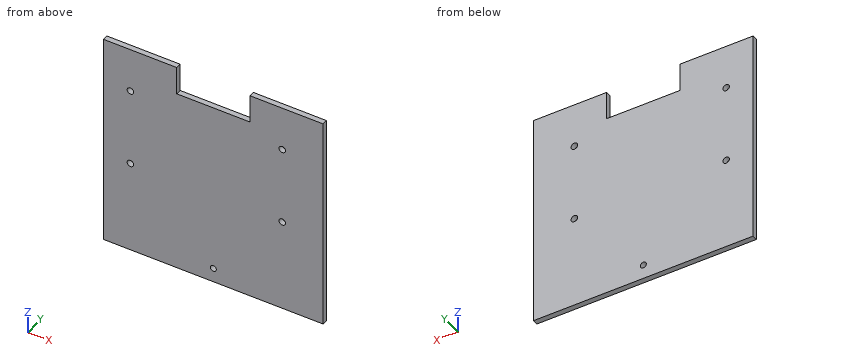
from build123d import *

# Parameters (mm, degrees)
SKETCH1_W           = 193.68
SKETCH1_H           = 190.5
BOSS_EXTRUDE1_DEPTH = 4.78
SKETCH2_R           = 2.6797
CUT_EXTRUDE1_DEPTH  = 5.78
CUT_EXTRUDE2_DEPTH  = 5.78
SKETCH4_R           = 2.893699953
CUT_EXTRUDE3_DEPTH  = 5.78


with BuildPart() as part:
    # Sketch1 → Boss-Extrude1 (new body)
    with BuildSketch(Plane(origin=(0, 0, 0), x_dir=(1, 0, 0), z_dir=(0, 1, 0))):
        Rectangle(SKETCH1_W, SKETCH1_H)
    extrude(amount=BOSS_EXTRUDE1_DEPTH)

    # Sketch2 → Cut-Extrude1 (cut, through all)
    with BuildSketch(Plane(origin=(0, 4.78, 0), x_dir=(1, 0, 0), z_dir=(0, 1, 0))):
        with Locations((0, 82.55)):
            Circle(SKETCH2_R)
    extrude(amount=-CUT_EXTRUDE1_DEPTH, mode=Mode.SUBTRACT)

    # Sketch3 → Cut-Extrude2 (cut, through all)
    with BuildSketch(Plane(origin=(0, 4.78, 0), x_dir=(1, 0, 0), z_dir=(0, 1, 0))):
        Polygon((0, -95.25), (-32.28, -95.25), (-32.28, -70.249999962), (32.28, -70.249999962), (32.28, -95.25), align=None)
    extrude(amount=-CUT_EXTRUDE2_DEPTH, mode=Mode.SUBTRACT)

    # Sketch4 → Cut-Extrude3 (cut, through all)
    with BuildSketch(Plane(origin=(0, 4.78, 0), x_dir=(1, 0, 0), z_dir=(0, 1, 0))):
        with Locations((-73.14, -55.899999962)):
            Circle(SKETCH4_R)
        with Locations((-73.14, 13.100000038)):
            Circle(SKETCH4_R)
        with Locations((60.86, 13.100000038)):
            Circle(SKETCH4_R)
        with Locations((60.86, -55.899999962)):
            Circle(SKETCH4_R)
    extrude(amount=-CUT_EXTRUDE3_DEPTH, mode=Mode.SUBTRACT)


solid = part.part
Input: part model. Units: mm. Frame: model coordinates. Coordinates: 2 decimals unless noted, no trailing zeros. Loops run counter-clockwise (first coordinate to the right, second up) from the corner with the lowest first, then second, coordinate; pieces in that order, holes last.
Q1. Contact query for a flat-ended pin moving along its axis: pin 1 (7 mm diameter, centred on x = 0, z = -82.55, fed in from -Y). Output: stop coordinate, or through.
Q2. Cut plane D-D (x = 0). Output: boundary loops of the cut face in (y, z).
Q3. Cut plane A-A (z = 55.9). Output: boundary loops of the cut face in (x, y).
Q4. Cut plane B-B (z = -82.55). Output: boundary loops of the cut face in (x, y).
Q5. Material intervals for line 1 (X direction, y = 3.05, z = 55.9); line 2 (Z direction, x = 60.86, y = 2.1); line 3 (Z direction, x = -71.5, y = 0.6), sorted ascending.
Q6. Cut plane C-C (y = 1.85). Output: boundary loops of the cut face in (x, z).
Working result:
1. pin 1: stops at y = 0
2. outline: (0, -95.25) - (4.78, -95.25) - (4.78, -85.23) - (0, -85.23) - close; (0, -79.87) - (4.78, -79.87) - (4.78, 70.25) - (0, 70.25) - close
3. outline: (-96.84, 0) - (-76.03, 0) - (-76.03, 4.78) - (-96.84, 4.78) - close; (-70.25, 0) - (57.97, 0) - (57.97, 4.78) - (-70.25, 4.78) - close; (63.75, 0) - (96.84, 0) - (96.84, 4.78) - (63.75, 4.78) - close
4. outline: (-96.84, 0) - (-2.68, 0) - (-2.68, 4.78) - (-96.84, 4.78) - close; (2.68, 0) - (96.84, 0) - (96.84, 4.78) - (2.68, 4.78) - close
5. line 1: x = -96.84 to -76.03, -70.25 to 57.97, 63.75 to 96.84
5. line 2: z = -95.25 to -15.99, -10.21 to 53.01, 58.79 to 95.25
5. line 3: z = -95.25 to -15.48, -10.72 to 53.52, 58.28 to 95.25
6. outline: (-96.84, -95.25) - (96.84, -95.25) - (96.84, 95.25) - (32.28, 95.25) - (32.28, 70.25) - (-32.28, 70.25) - (-32.28, 95.25) - (-96.84, 95.25) - close; hole circle Ø5.79 at (-73.14, -13.1); hole circle Ø5.79 at (-73.14, 55.9); hole circle Ø5.36 at (0, -82.55); hole circle Ø5.79 at (60.86, -13.1); hole circle Ø5.79 at (60.86, 55.9)
